Read the model definition and answer for the solid it produces. Units are mm, in the model's axes. Give positions to 0.01 mm unless a question says otherwise; leave off trailing zeros. Loops run counter-clockwise (first coordinate to the right, second up) from the corner with the lowest first, then second, coordinate; pieces in that order, holes last.
(1) Determine the mould class of faces 1 (the face through (-85, 0, 2)), 2 (the face through (-25.593, -13.563, 2.465)), 3 (the face through (-32, 0, 5)), 4 (the face through (-0.195, -13.413, 2.465)) for opening direction X: pulls with the +X half, pulls with the -X half, needs draft (parallel to the pull), parting line crosses it, or undercut.
(2) Find section D-D, the plane x = -70. Write down the section's boundary in (y, z).
(3) Each of these flat-tipped pins is pushed along its axis until it touches: P1, Ø6, axis at x = -21.5, y = 14, coming from the -Z side; P2, Ø1.5, axis at x = -1.5, z = 2, coming from the -Y side; P3, Ø3, axis at y = -5, z = 4, coming from the -X side; P4, Ø1, axis at y = -5, z = 0.5, coming from the +X side. Where does it stop, or does it pass through?
(4) Find section A-A, the plane x = 0. Write down the section's boundary in (y, z).
(5) Find section B-B, the plane y = 0. Write down the section's boundary in (x, z).
(6) Find section C-C, the plane z = 2.8. Write down the section's boundary in (x, y).
(7) Straight lines are drawn through the part: probe 1 along Y at (x, z) = (0, 3.6); probe 2 along X at (y, z) = (2, 0.9); probe 3 along X at (y, z) = (7.5, 2.4). For each, find the intervals that lie inside material, in ascending order.
```python
from build123d import *

# Parameters (mm, degrees)
SKETCH1_R           = 7
SKETCH1_R_2         = 10
SKETCH1_R_3         = 1.5
SKETCH1_R_4         = 1.75
BOSS_EXTRUDE1_DEPTH = 5


with BuildPart() as part:
    # Sketch1 → Boss-Extrude1 (new body)
    with BuildSketch(Plane.XY):
        with BuildLine():
            Line((-71.071428571, 14.961685761), (-1.428571429, 19.948914348))
            ThreePointArc((-1.428571429, 19.948914348), (20, 0), (-1.428571429, -19.948914348))
            Line((-1.428571429, -19.948914348), (-71.071428571, -14.961685761))
            ThreePointArc((-71.071428571, -14.961685761), (-85, 0), (-71.071428571, 14.961685761))
        make_face()
        with Locations((-70, 0)):
            Circle(SKETCH1_R, mode=Mode.SUBTRACT)
        Circle(SKETCH1_R_2, mode=Mode.SUBTRACT)
        with Locations((-12.903778516, 7.45)):
            Circle(SKETCH1_R_3, mode=Mode.SUBTRACT)
        with Locations((0, -14.9)):
            Circle(SKETCH1_R_3, mode=Mode.SUBTRACT)
        with Locations((-27.262321561, 14.088677781)):
            Circle(SKETCH1_R_4, mode=Mode.SUBTRACT)
        with Locations((-27.262321561, -14.088677781)):
            Circle(SKETCH1_R_4, mode=Mode.SUBTRACT)
        with Locations((12.903778516, 7.45)):
            Circle(SKETCH1_R_3, mode=Mode.SUBTRACT)
    extrude(amount=BOSS_EXTRUDE1_DEPTH)


solid = part.part
```
Entries:
1. face 1: pulls with the -X half
1. face 2: undercut
1. face 3: needs draft
1. face 4: undercut
2. outline: (-15.04, 0) - (-7, 0) - (-7, 5) - (-15.04, 5) - close; (7, 0) - (15.04, 0) - (15.04, 5) - (7, 5) - close
3. P1: stops at z = 0
3. P2: stops at y = -19.99
3. P3: stops at x = -84.59
3. P4: stops at x = 19.49
4. outline: (-20, 0) - (-16.4, 0) - (-16.4, 5) - (-20, 5) - close; (-13.4, 0) - (-10, 0) - (-10, 5) - (-13.4, 5) - close; (10, 0) - (20, 0) - (20, 5) - (10, 5) - close
5. outline: (-85, 0) - (-77, 0) - (-77, 5) - (-85, 5) - close; (-63, 0) - (-10, 0) - (-10, 5) - (-63, 5) - close; (10, 0) - (20, 0) - (20, 5) - (10, 5) - close
6. outline: (-71.07, -14.96) - (-1.43, -19.95) arc R20 ccw (long way) to (-1.43, 19.95) - (-71.07, 14.96) arc R15 ccw to start; hole circle Ø14 at (-70, 0); hole circle Ø3.5 at (-27.26, -14.09); hole circle Ø3.5 at (-27.26, 14.09); hole circle Ø3 at (-12.9, 7.45); hole circle Ø20 at (0, 0); hole circle Ø3 at (0, -14.9); hole circle Ø3 at (12.9, 7.45)
7. probe 1: y = -20 to -16.4, -13.4 to -10, 10 to 20
7. probe 2: x = -84.87 to -76.71, -63.29 to -9.8, 9.8 to 19.9
7. probe 3: x = -82.99 to -14.4, -11.4 to -6.61, 6.61 to 11.4, 14.4 to 18.54
